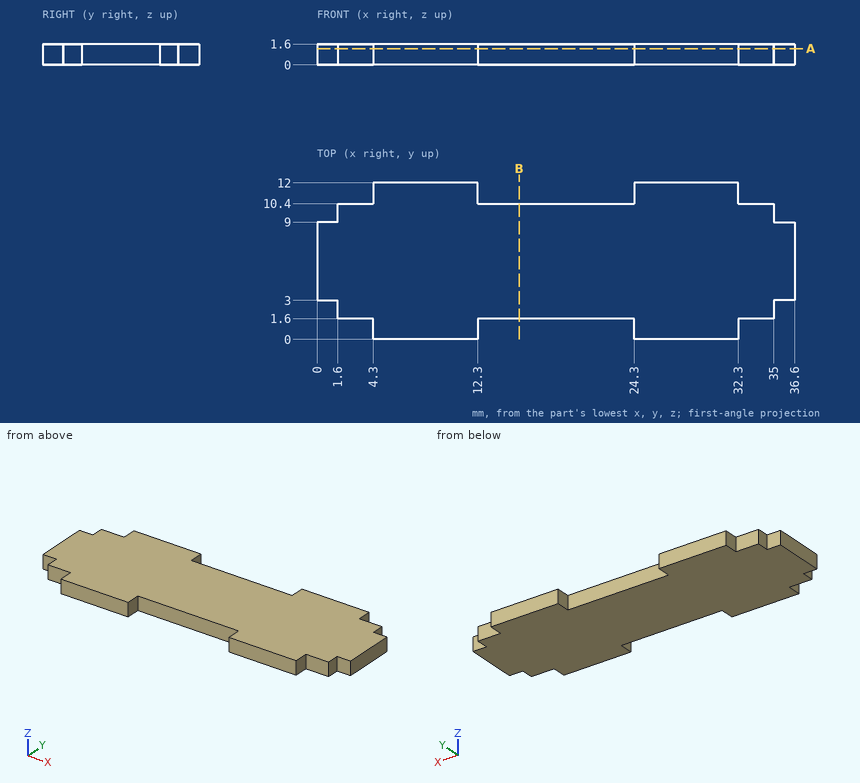
For this review, use the dimensioned drawing (mm, ordinates from the lowest corner) and the shaded views. Coordinates: 2 decimals unless noted, no trailing zeros. Order: outer loops, then holes, each group sorted by start corner. A loop starts at its lowest first (then second) coordinate and runs counter-clockwise, first axis right, second up. Notation, with made-up numbers: (-19, -26.5) - (23, -26.5) arc R7 cw to (23, -15.5) - close; hole circle Ø8 at (-39.5, -27.5). An arc over 180 degrees is marked (long way). Answer as a JSON object with one key per item and string values. Group by question number.
1. Clearance check with flat-ended pins moving along their axes: P1, Ø0.5, axis at x = 3, z = 0.5, coming from the +Y side; P2, Ø0.5, axis at x = 35.5, z = 1, coming from the +Y side; P3, Ø0.8, axis at y = 11.5, z = 1, coming from the +X side. State where each tip first meets the part, or that it passes through.
2. We need section B-B on x = 15.5. State the section outline as (y, z) points, then the cut area to 3 significant figures.
3. We need section A-A on z = 1.25. State the section outline as (x, y) points.
4. For probe 1 along X at (y, z) = (1, 0.1); probe 2 along Y at (x, z) = (21, 0.1); probe 3 along X at (y, z) = (2.5, 0.45), list the stretches that pass through material, from the lowest coordinate up.
Final values:
{
 "1": {"P1": "y = 10.4", "P2": "y = 9", "P3": "x = 32.3"},
 "2": {"outline": "(1.6, 0) - (10.4, 0) - (10.4, 1.6) - (1.6, 1.6) - close", "area": "14.1 mm²"},
 "3": {"outline": "(0, 3) - (1.6, 3) - (1.6, 1.6) - (4.3, 1.6) - (4.3, 0) - (12.3, 0) - (12.3, 1.6) - (24.3, 1.6) - (24.3, 0) - (32.3, 0) - (32.3, 1.6) - (35, 1.6) - (35, 3) - (36.6, 3) - (36.6, 9) - (35, 9) - (35, 10.4) - (32.3, 10.4) - (32.3, 12) - (24.3, 12) - (24.3, 10.4) - (12.3, 10.4) - (12.3, 12) - (4.3, 12) - (4.3, 10.4) - (1.6, 10.4) - (1.6, 9) - (0, 9) - close"},
 "4": {"probe 1": "4.3 to 12.3, 24.3 to 32.3", "probe 2": "1.6 to 10.4", "probe 3": "1.6 to 35"}
}
